from build123d import *

# Parameters (mm, degrees)
SKETCH1_R                = 26
BOSS_EXTRUDE1_DEPTH      = 40
SKETCH2_R                = 11.25
F_608_BEARING_HOLE_DEPTH = 7.5
SKETCH3_R                = 6.75
F_624_BEARING_HOLE_DEPTH = 5.5
SKETCH4_R                = 2
CUT_EXTRUDE3_DEPTH       = 41


with BuildPart() as part:
    # Sketch1 → Boss-Extrude1 (new body)
    with BuildSketch(Plane(origin=(0, 0, 0), x_dir=(1, 0, 0), z_dir=(0, 1, 0))):
        Circle(SKETCH1_R)
    extrude(amount=BOSS_EXTRUDE1_DEPTH)

    # Sketch2 → 608_Bearing_Hole (cut)
    with BuildSketch(Plane.XZ):
        Circle(SKETCH2_R)
    extrude(amount=-F_608_BEARING_HOLE_DEPTH, mode=Mode.SUBTRACT)

    # Sketch3 → 624_Bearing_Hole (cut)
    with BuildSketch(Plane(origin=(0, 40, 0), x_dir=(1, 0, 0), z_dir=(0, 1, 0))):
        Circle(SKETCH3_R)
    extrude(amount=-F_624_BEARING_HOLE_DEPTH, mode=Mode.SUBTRACT)

    # Sketch4 → Cut-Extrude3 (cut, through all)
    with BuildSketch(Plane(origin=(0, 40, 0), x_dir=(1, 0, 0), z_dir=(0, 1, 0))):
        Circle(SKETCH4_R)
    extrude(amount=-CUT_EXTRUDE3_DEPTH, mode=Mode.SUBTRACT)

    # Sketch5 → Cut-Revolve1 (revolve, cut)
    with BuildSketch(Plane(origin=(0, 0, 0), x_dir=(0, 0, -1), z_dir=(1, 0, 0))):
        Polygon((-26, 16), (-26, 24), (-18, 22.5), (-18, 17.5), align=None)
    revolve(axis=Axis((0, 0, 0), (0, 1, 0)), mode=Mode.SUBTRACT)


solid = part.part
The listing builds one solid part. Answer for the finished solid, in the listing's coordinates (mm). A direction names the side the tool comes from. Give positions to 0.01 mm unless a question says otherwise; leave off trailing zeros. Loops run counter-clockwise (first coordinate to the right, second up) from the corner with the lowest first, then second, coordinate; pieces in that order, holes last.
Item 1: Find the intervals of material crossed by line 1 along Y through (x, z) = (15, -10); line 2 along X through (y, z) = (38, 0); line 3 along Z through (x, y) = (0, 4), in increasing order.
Derived:
line 1: y = 0 to 17.49, 22.51 to 40
line 2: x = -26 to -6.75, 6.75 to 26
line 3: z = -26 to -11.25, 11.25 to 26
Item 2: A cutting plane is placed at C-C (y = 19). Give the vertices of the cut face in (x, z), then the cut area to 3 significant figures.
Derived:
outline: circle Ø36 at (0, 0); hole circle Ø4 at (0, 0)
area: 1,010 mm2
Item 3: A cutting plane is placed at D-D (y = 31.5). Give the vertices of the cut face in (x, z).
Derived:
outline: circle Ø52 at (0, 0); hole circle Ø4 at (0, 0)
Item 4: A cutting plane is placed at A-A (z = 0). Give the vertices of the cut face in (x, y).
Derived:
outline: (-26, 0) - (-11.25, 0) - (-11.25, 7.5) - (-2, 7.5) - (-2, 34.5) - (-6.75, 34.5) - (-6.75, 40) - (-26, 40) - (-26, 24) - (-18, 22.5) - (-18, 17.5) - (-26, 16) - close; (2, 7.5) - (11.25, 7.5) - (11.25, 0) - (26, 0) - (26, 16) - (18, 17.5) - (18, 22.5) - (26, 24) - (26, 40) - (6.75, 40) - (6.75, 34.5) - (2, 34.5) - close
Item 5: Each of these flat-tipped pins is pushed along its axis until it touches: pin 1 Ø12 at (x, y) = (18, 29) entering from +Z; pin 2 Ø3 at (x, z) = (0, 0) entering from +Y; pin 3 Ø3 at (y, z) = (34.5, -16) entering from +X; pin 4 Ø17.5 at (x, z) = (0, 0) entering from -Y. Where does it stop, or does it pass through?
Derived:
pin 1: stops at z = 23.07
pin 2: passes through
pin 3: stops at x = 21.58
pin 4: stops at y = 7.5
Item 6: A cutting plane is placed at B-B (x = 0). Give the vertices of the cut face in (y, z), then the cut area to 4 significant figures.
Derived:
outline: (0, -26) - (16, -26) - (17.5, -18) - (22.5, -18) - (24, -26) - (40, -26) - (40, -6.75) - (34.5, -6.75) - (34.5, -2) - (7.5, -2) - (7.5, -11.25) - (0, -11.25) - close; (0, 11.25) - (7.5, 11.25) - (7.5, 2) - (34.5, 2) - (34.5, 6.75) - (40, 6.75) - (40, 26) - (24, 26) - (22.5, 18) - (17.5, 18) - (16, 26) - (0, 26) - close
area: 1,625 mm2
Item 7: Determine the mould class of faces 1 (the flat face through (1, 34.5, -2)), 2 (the conical face through (5.557, 17.406, 17.646)), 3 (the flat face through (5, 40, 5)) for opening direction Z: +Z half, -Z half, draft (parallel to the pull), parting line (faces both ways), or undercut.
Derived:
face 1: undercut
face 2: parting line
face 3: draft
Item 8: A tool of negligible diameter and unlimited length cuts with its end or side. For faces 4 (the cylindrical face through (-1.46, 37.29, 6.59)), 5 (the cylindrical face through (5.19, 3.7, -9.98)), 6 (the cylindrical face through (17.847, 19.965, -2.343)), from which of +Z, -Z, +X, -X, +Y, -Y can it reach the whole face along a straight path? Write none if from no direction.
Derived:
face 4: +Y
face 5: -Y
face 6: none
